Verification items for the finished model (mm, model axes). Face numbers are marked on the shaded views. A direction names the side the tool comes from. Coordinates: 2 decimals unless noted, no trailing zeros. Order: outer loops, then holes, each group sorted by start corner. A loop starts at its lowest first (then second) coordinate and runs counter-clockwise, first axis right, second up. Notation, with made-up numbers: M 81.5,51 L 98.5,51 A34 cw 98.5,84 Z; hole C 0,51.5 d1. An arc over 180 degrees is marked long. Use one line per item in the form item = value. Start each with the question number.
```python
from build123d import *

# Parameters (mm, degrees)
SKETCH1_W                       = 25.4
SKETCH1_H                       = 50.8
BOSS_EXTRUDE1_DEPTH             = 3.175
F_10_CLEARANCE_HOLE1_D          = 5.6134
BOSS_EXTRUDE3_DEPTH             = 31.75
CHAMFER2_SIZE                   = 12.7
FILLET2_R                       = 0.635
BOSS_EXTRUDE4_REACH             = 64.331
BOSS_EXTRUDE4_DIRECTION_2_DEPTH = 3.175
BOSS_EXTRUDE5_REACH             = 64.331
BOSS_EXTRUDE5_DIRECTION_2_DEPTH = 3.175
F_1_4_CLEARANCE_HOLE2_REACH     = 70.01
F_1_4_CLEARANCE_HOLE2_BORE_R    = 3.57124
CUT_EXTRUDE1_START              = -9.525
CUT_EXTRUDE1_DEPTH              = 19.05


# Read off the part's stored shape, not the designer's step: Cut-Extrude1
with BuildPart() as part:
    # Sketch1 → Boss-Extrude1 (new body)
    with BuildSketch(Plane.XY):
        Rectangle(SKETCH1_W, SKETCH1_H)
    extrude(amount=BOSS_EXTRUDE1_DEPTH)

    # #10 Clearance Hole1 (through all)
    with Locations(Plane(origin=(0, 0, 0), x_dir=(-1, 0, 0), z_dir=(0, 0, -1))):
        with Locations((0, 12.7), (0, -12.7)):
            Hole(F_10_CLEARANCE_HOLE1_D / 2)

    # Sketch8 → Boss-Extrude3 (add, symmetric)
    with BuildSketch(Plane(origin=(0, 0, 0), x_dir=(0, 0, -1), z_dir=(1, 0, 0))):
        Polygon((0, 33.90738686), (-31.75, 25.4), (0, 25.4), align=None)
    extrude(amount=BOSS_EXTRUDE3_DEPTH, both=True)

    # Chamfer2
    chamfer2_edges = [part.edges().sort_by_distance(p)[0] for p in [
        (-12.7, 25.4, 1.5875),
        (12.7, 25.4, 1.5875),
    ]]
    chamfer(chamfer2_edges, length=CHAMFER2_SIZE)

    # Fillet2
    fillet2_edges = [part.edges().sort_by_distance(p)[0] for p in [
        (0, 25.4, 31.75),
    ]]
    fillet(fillet2_edges, radius=FILLET2_R)

    # Boss-Extrude4: up to this face of the body (flat: up to its plane)
    boss_extrude4_end = Plane(part.part.faces().sort_by_distance((-19.05, 19.05, 1.5875))[0])
    # Sketch14 → Boss-Extrude4 (add, up to the picked face)
    with BuildSketch(Plane.ZY.offset(12.7), mode=Mode.PRIVATE) as boss_extrude4_sk1:
        Polygon((3.175, 12.7), (15.875, 25.4), (3.175, 25.4), align=None)
    boss_extrude4_tool1 = split(extrude(boss_extrude4_sk1.sketch, amount=BOSS_EXTRUDE4_REACH, mode=Mode.PRIVATE), bisect_by=boss_extrude4_end, keep=Keep.BOTH, mode=Mode.PRIVATE)
    add(boss_extrude4_tool1.solids().sort_by(Axis((-12.7, 21.166667, 7.408333), (-1, 0, 0)))[0])

    # Sketch14 → Boss-Extrude4 direction 2 (add)
    with BuildSketch(Plane.ZY.offset(12.7)):
        Polygon((3.175, 12.7), (15.875, 25.4), (3.175, 25.4), align=None)
    extrude(amount=-BOSS_EXTRUDE4_DIRECTION_2_DEPTH)

    # Boss-Extrude5: up to this face of the body (flat: up to its plane)
    boss_extrude5_end = Plane(part.part.faces().sort_by_distance((19.05, 19.05, 1.5875))[0])
    # Sketch15 → Boss-Extrude5 (add, up to the picked face)
    with BuildSketch(Plane(origin=(12.7, 0, 0), x_dir=(0, 0, -1), z_dir=(1, 0, 0)), mode=Mode.PRIVATE) as boss_extrude5_sk1:
        Polygon((-3.175, 12.7), (-15.875, 25.4), (-3.175, 25.4), align=None)
    boss_extrude5_tool1 = split(extrude(boss_extrude5_sk1.sketch, amount=BOSS_EXTRUDE5_REACH, mode=Mode.PRIVATE), bisect_by=boss_extrude5_end, keep=Keep.BOTH, mode=Mode.PRIVATE)
    add(boss_extrude5_tool1.solids().sort_by(Axis((12.7, 21.166667, 7.408333), (1, 0, 0)))[0])

    # Sketch15 → Boss-Extrude5 direction 2 (add)
    with BuildSketch(Plane(origin=(12.7, 0, 0), x_dir=(0, 0, -1), z_dir=(1, 0, 0))):
        Polygon((-3.175, 12.7), (-15.875, 25.4), (-3.175, 25.4), align=None)
    extrude(amount=-BOSS_EXTRUDE5_DIRECTION_2_DEPTH)

    # 1/4 Clearance Hole2 bore → 1/4 Clearance Hole2 (cut, up to next)
    with BuildSketch(Plane(origin=(0, 31.636022628, 8.476846715), x_dir=(1, 0, 0), z_dir=(0, 0.96592582628907, 0.2588190451025146)), mode=Mode.PRIVATE) as f_1_4_clearance_hole2_sk1:
        with Locations((0, -3.924122511)):
            Circle(F_1_4_CLEARANCE_HOLE2_BORE_R)
    f_1_4_clearance_hole2_tool1 = extrude(f_1_4_clearance_hole2_sk1.sketch, amount=-F_1_4_CLEARANCE_HOLE2_REACH, mode=Mode.PRIVATE) & part.part
    add(f_1_4_clearance_hole2_tool1.solids().sort_by_distance((0, 30.620385, 12.267258))[0], mode=Mode.SUBTRACT)

    # Cut-Extrude1 outline → Cut-Extrude1 (cut)
    with BuildSketch(Plane.YZ.offset(CUT_EXTRUDE1_START)):
        Polygon((29.112245926, 3.175), (25.4, 17.029290407), (25.4, 3.175), align=None)
    extrude(amount=CUT_EXTRUDE1_DEPTH, mode=Mode.SUBTRACT)


solid = part.part
```
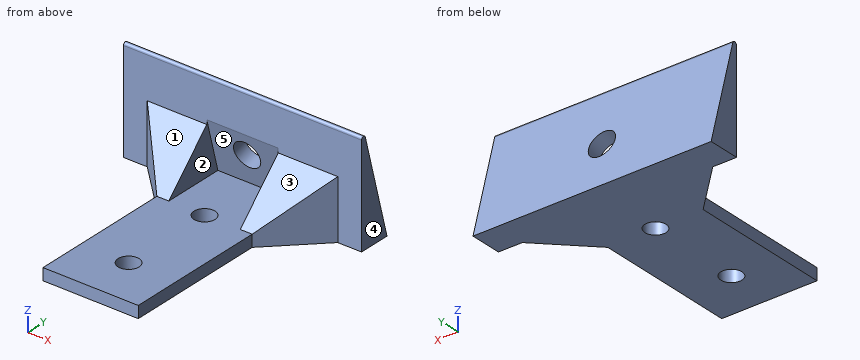
1. Cross-section at D-D on y = 24. Enter the section's corners in (x, z) (3 decimals), and give its area (3 significant figures).
2. Release check for a two-part mould opening along Z. For the marked faces 3, 4 and 5 record: pulls with the +Z half, pulls with the -Z half, needs draft (parallel to the pull), parting line crosses it, or undercut.
3. Tool access check on the marked faces 1 and 2. Record the directions out of +Z, -Z, +X, -X, +Y, -Y that give a thin tool (end or side, any length) a straight path to the whole face; none if there is none.
4. Material ranges on line 1 along Y through (x, z) = (0, 2.25); line 2 along Y through (x, z) = (0, 1.4); line 3 along Z through (x, y) = (-5, -3) (3 decimals), recorded low to high.
5. Cross-section at B-B on x = 0. Enter the section's corners in (y, z) (3 decimals), and give its area (3 significant figures).
6. Depth check by flat-ended pin: P1, Ø15, axis at y = 22, z = 7, coming from the +X side; P2, Ø12, axis at x = -10.5, z = 8, coming from the +Y side; P3, Ø8, axis at x = -4.5, z = 20.5, coming from the +Y side; P4, Ø7.5, axis at x = 1, y = -10.5, coming from the +Z side (3 decimals). Enter the tip coordinate at first touch or a pass-through.
7. Cross-section at C-C on z = 6.25. Enter the section's corners in (x, y) (3 decimals).
8. Cross-section at A-A on y = -12.7. Enter the section's corners in (x, z) (3 decimals).
Final values:
q1.outline = M -24,0 L 24,0 L 24,14.475 L 9.525,14.475 L 9.525,3.175 L -9.525,3.175 L -9.525,14.475 L -24,14.475 Z
q1.area = 480 mm2
q2.face_3 = pulls with the +Z half
q2.face_4 = needs draft
q2.face_5 = undercut
q3.face_1 = +Z, +X, -X, -Y
q3.face_2 = -Y
q4.line_1 = -25.4 to -15.51, -9.89 to 9.89, 15.51 to 33.3
q4.line_2 = -25.4 to -15.51, -9.89 to 9.89, 15.51 to 33.53
q4.line_3 = 0 to 3.175
q5.outline = M -25.4,0 L -15.507,0 L -15.507,3.175 L -25.4,3.175 Z; M -9.893,0 L 9.893,0 L 9.893,3.175 L -9.893,3.175 Z; M 15.507,0 L 33.907,0 L 31.545,8.818 L 27.865,7.832 L 29.112,3.175 L 15.507,3.175 Z; M 25.4,17.029 L 26.016,14.731 L 29.696,15.717 L 26.648,27.091 A0.635 ccw 25.4,26.927 Z
q5.area = 205 mm2
q6.P1 = 31.75
q6.P2 = 33.37
q6.P3 = 29.49
q6.P4 = 3.175
q7.outline = M -31.75,25.4 L -25.4,25.4 L -15.775,15.775 L -9.525,15.775 L -9.525,28.288 L 9.525,28.288 L 9.525,15.775 L 15.775,15.775 L 25.4,25.4 L 31.75,25.4 L 31.75,32.233 L -31.75,32.233 Z
q8.outline = M -12.7,0 L -2.807,0 L -2.807,3.175 L -12.7,3.175 Z; M 2.807,0 L 12.7,0 L 12.7,3.175 L 2.807,3.175 Z
